Check sheet for the modelled part. Datum: model origin and axes. Units: mm. Coordinates: 2 decimals unless noted, no trailing zeros. Loops run counter-clockwise (first coordinate to the right, second up) from the corner with the lowest first, then second, coordinate; pieces in that order, holes last. Notation, with made-up numbers: (7, 19) - (30, 19) arc R30 cw to (30, 46) - close; hole circle Ø11 at (-38.75, -14.75). An arc over 180 degrees is marked (long way). Use a Markdown table: item, result. Add a question column.
1) Sectioned sample at C-C, the plane x = -2. Enter the section's corners in (y, z), then the cut area to 3 significant figures.
2) Go/stop test with flat-tipped pins: P1, Ø5.5, axis at y = 29, z = 12, coming from the +X side; P2, Ø1, axis at y = 16, z = 13, coming from the -X side; P3, Ø1, axis at x = 3, y = -10.5, coming from the -Z side; P4, Ø2.5, axis at x = 4, z = -24.5, coming from the -Y side. Record where each tip stops, or that it passes through.
3) Sectioned sample at A-A, the plane z = 67. State how many separate pieces and enclosed holes the cut face has, then the cut area to 3 significant figures.
4) Thickness scan on line 1 (Z direction, x = 3.75, y = 5.5); line 2 (Z direction, x = 5.5, y = 4.5); line 3 (X direction, y = -8.5, z = 6). Record the ranges inside material, lowest first.
5) Sectioned sample at B-B, the plane y = -2. Enter the section's corners in (x, z).
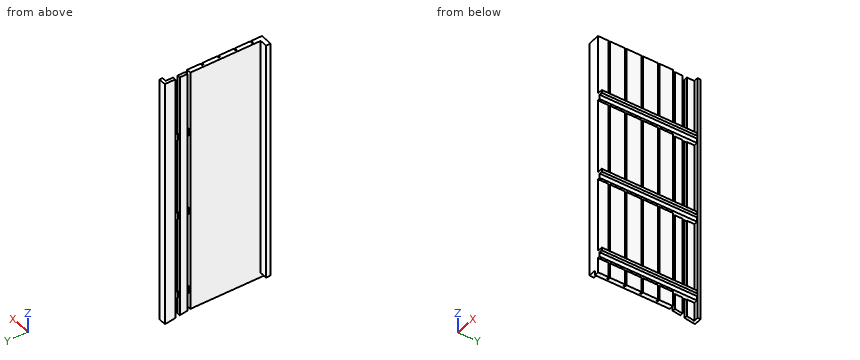
from build123d import *

# Parameters (mm, degrees)
SKETCH1_W           = 165
SKETCH1_H           = 50
BOSS_EXTRUDE1_DEPTH = 3
SKETCH3_W           = 165
SKETCH3_H           = 1
CUT_EXTRUDE1_DEPTH  = 1.5
SKETCH4_W           = 5
SKETCH4_H           = 65
BOSS_EXTRUDE2_DEPTH = 1.5
SKETCH5_W           = 2
SKETCH5_H           = 65
BOSS_EXTRUDE3_DEPTH = 2
FILLET1_R           = 2
SKETCH8_W           = 167.5
SKETCH8_H           = 5
BOSS_EXTRUDE4_DEPTH = 2
SKETCH6_W           = 5
SKETCH6_H           = 167.5
BOSS_EXTRUDE5_DEPTH = 2
CUT_EXTRUDE2_DEPTH  = 3
SKETCH10_W          = 165
SKETCH10_H          = 3
BOSS_EXTRUDE6_DEPTH = 5
SKETCH11_W          = 5
SKETCH11_H          = 3
CUT_EXTRUDE3_DEPTH  = 3


with BuildPart() as part:
    # Sketch1 → Boss-Extrude1 (new body)
    with BuildSketch(Plane(origin=(0, 0, 0), x_dir=(0, 0, -1), z_dir=(1, 0, 0))):
        Rectangle(SKETCH1_W, SKETCH1_H)
    extrude(amount=BOSS_EXTRUDE1_DEPTH)

    # Sketch3 → Cut-Extrude1 (cut)
    with BuildSketch(Plane(origin=(3, 0, 0), x_dir=(0, 0, -1), z_dir=(1, 0, 0))):
        with Locations((0, -17.5)):
            Rectangle(SKETCH3_W, SKETCH3_H)
        with Locations((0, -6.5)):
            Rectangle(SKETCH3_W, SKETCH3_H)
        with Locations((0, 4.5)):
            Rectangle(SKETCH3_W, SKETCH3_H)
        with Locations((0, 15.5)):
            Rectangle(SKETCH3_W, SKETCH3_H)
    extrude(amount=-CUT_EXTRUDE1_DEPTH, mode=Mode.SUBTRACT)

    # Sketch4 → Boss-Extrude2 (add, symmetric)
    with BuildSketch(Plane(origin=(3, 0, 0), x_dir=(0, 0, -1), z_dir=(1, 0, 0))):
        with Locations((-40, 7.5)):
            Rectangle(SKETCH4_W, SKETCH4_H)
        with Locations((15, 7.5)):
            Rectangle(SKETCH4_W, SKETCH4_H)
        with Locations((70, 7.5)):
            Rectangle(SKETCH4_W, SKETCH4_H)
    extrude(amount=BOSS_EXTRUDE2_DEPTH, both=True)

    # Sketch5 → Boss-Extrude3 (add)
    with BuildSketch(Plane(origin=(4.5, 0, 0), x_dir=(0, 0, -1), z_dir=(1, 0, 0))):
        with Locations((-41.5, 7.5)):
            Rectangle(SKETCH5_W, SKETCH5_H)
        with Locations((13.5, 7.5)):
            Rectangle(SKETCH5_W, SKETCH5_H)
        with Locations((68.5, 7.5)):
            Rectangle(SKETCH5_W, SKETCH5_H)
    extrude(amount=BOSS_EXTRUDE3_DEPTH)

    # Fillet1
    fillet1_edges = [part.edges().sort_by_distance(p)[0] for p in [
        (6.5, 40, -68.5),
        (6.5, 40, -13.5),
        (6.5, 40, 41.5),
    ]]
    fillet(fillet1_edges, radius=FILLET1_R)

    # Sketch8 → Boss-Extrude4 (add)
    with BuildSketch(Plane.ZY):
        with Locations((-1.25, 37.5)):
            Rectangle(SKETCH8_W, SKETCH8_H)
        with Locations((-1.25, 29.5)):
            Rectangle(SKETCH8_W, SKETCH8_H)
    extrude(amount=-BOSS_EXTRUDE4_DEPTH)

    # Sketch6 → Boss-Extrude5 (add)
    with BuildSketch(Plane(origin=(0, 40, 0), x_dir=(1, 0, 0), z_dir=(0, 1, 0))):
        with Locations((2.5, 1.25)):
            Rectangle(SKETCH6_W, SKETCH6_H)
    extrude(amount=BOSS_EXTRUDE5_DEPTH)

    # Sketch9 → Cut-Extrude2 (cut)
    with BuildSketch(Plane(origin=(3, 0, 0), x_dir=(0, 0, -1), z_dir=(1, 0, 0))):
        Polygon((82.5, 25), (85, 40), (86.823403956, 40), (86.823403956, 25), align=None)
    extrude(amount=-CUT_EXTRUDE2_DEPTH, mode=Mode.SUBTRACT)

    # Sketch10 → Boss-Extrude6 (add)
    with BuildSketch(Plane.ZY):
        with Locations((0, -23.5)):
            Rectangle(SKETCH10_W, SKETCH10_H)
    extrude(amount=BOSS_EXTRUDE6_DEPTH)

    # Sketch11 → Cut-Extrude3 (cut)
    with BuildSketch(Plane(origin=(0, -22, 0), x_dir=(1, 0, 0), z_dir=(0, 1, 0))):
        with Locations((-2.5, 81)):
            Rectangle(SKETCH11_W, SKETCH11_H)
    extrude(amount=-CUT_EXTRUDE3_DEPTH, mode=Mode.SUBTRACT)


solid = part.part
Solved:
| question | item | result |
|---|---|---|
| 1 | outline | (-25, -79.5) - (-22, -79.5) - (-22, 82.5) - (-25, 82.5) - close |
| 1 | area | 486 mm2 |
| 2 | P1 | stops at x = 2 |
| 2 | P2 | stops at x = 0 |
| 2 | P3 | stops at z = -82.5 |
| 2 | P4 | stops at y = -25 |
| 3 | separate pieces | 3 |
| 3 | enclosed holes | 0 |
| 3 | area | 189 mm2 |
| 4 | line 1 | z = -72.5 to -67.5, -17.5 to -12.5, 37.5 to 42.5 |
| 4 | line 2 | z = -69.5 to -67.5, -14.5 to -12.5, 40.5 to 42.5 |
| 4 | line 3 | x = 0 to 3 |
| 5 | outline | (0, -82.5) - (3, -82.5) - (3, -72.5) - (4.5, -72.5) - (4.5, -69.5) - (6.5, -69.5) - (6.5, -67.5) - (3, -67.5) - (3, -17.5) - (4.5, -17.5) - (4.5, -14.5) - (6.5, -14.5) - (6.5, -12.5) - (3, -12.5) - (3, 37.5) - (4.5, 37.5) - (4.5, 40.5) - (6.5, 40.5) - (6.5, 42.5) - (3, 42.5) - (3, 82.5) - (0, 82.5) - close |
